from build123d import *

# Parameters (mm, degrees)
F0_R      = 15.625
F1_DEPTH  = 4
F2_R      = 2.45
F3_DEPTH  = 2
F4_R      = 3
F5_DEPTH  = 9.1
F6_R      = 1.55
F7_DEPTH  = 6
F8_R      = 5.5
F9_DEPTH  = 1
F11_R     = 0.5
F12_DEPTH = 1
F13_R     = 2
F14_DEPTH = 25.4


# Not quite as in the source:
# - a fillet or chamfer that OpenCascade refuses, or shapes differently, is made with other operations: its cross-section is extruded or revolved along the edge and cut away or added


with BuildPart() as f1:
    # F0 (on Front) → F1 (new body)
    with BuildSketch(Plane.XZ):
        Circle(F0_R)
    extrude(amount=F1_DEPTH)

    # F2 (on face) → F3 (join)
    with BuildSketch(Plane.XZ.offset(4)):
        Circle(F2_R)
    extrude(amount=F3_DEPTH)

    # F4 (on face) → F5 (join)
    with BuildSketch(Plane(origin=(0, 0, 0), x_dir=(-1, 0, 0), z_dir=(0, 1, 0))):
        Circle(F4_R)
    extrude(amount=F5_DEPTH)

    # F6 (on face) → F7 (cut)
    with BuildSketch(Plane(origin=(0, 9.1, 0), x_dir=(-1, 0, 0), z_dir=(0, 1, 0))):
        Circle(F6_R)
    extrude(amount=-F7_DEPTH, mode=Mode.SUBTRACT)

    # F8 (on face) → F9 (join)
    with BuildSketch(Plane.XZ.offset(4)):
        Circle(F8_R)
    extrude(amount=F9_DEPTH)

    # F10: fillet of radius 1.5875 on 3 edges, made by hand

    # F10_s1 → F10_t2 (revolve, cut)
    with BuildSketch(Plane.XY):
        with BuildLine():
            ThreePointArc((15.625, -2.4125), (15.1600320151, -3.5350320151), (14.0375, -4))
            Line((14.0375, -4), (15.625, -4))
            Line((15.625, -4), (15.625, -2.4125))
        make_face()
    revolve(axis=Axis((0, -4, 0), (0, -1, 0)), mode=Mode.SUBTRACT)

    # F10_s3 → F10_t4 (revolve, cut)
    with BuildSketch(Plane.XY):
        with BuildLine():
            ThreePointArc((15.625, -1.5875), (15.1600320151, -0.4649679849), (14.0375, 0))
            Line((14.0375, 0), (15.625, 0))
            Line((15.625, 0), (15.625, -1.5875))
        make_face()
    revolve(axis=Axis((0, 0, 0), (0, -1, 0)), mode=Mode.SUBTRACT)

    # F10_s5 → F10_t6 (revolve, cut)
    with BuildSketch(Plane.XY):
        with BuildLine():
            ThreePointArc((5.5, -4), (4.9161383637, -4.7264277948), (4.0252118796, -5))
            Line((4.0252118796, -5), (5.5, -5))
            Line((5.5, -5), (5.5, -4))
        make_face()
    revolve(axis=Axis((0, -5, 0), (0, -1, 0)), mode=Mode.SUBTRACT)

    # F11 (on face) → F12 (join)
    with BuildSketch(Plane.XZ.offset(5)):
        with Locations((-2.9818608891, 0.9871639777)):
            Circle(F11_R)
        with Locations((-2.258730121, 2.6503647678)):
            Circle(F11_R)
        with Locations((1.9354285905, 2.7226777747)):
            Circle(F11_R)
        with Locations((3.0201247428, 0.9510074742)):
            Circle(F11_R)
        with Locations((2.0800547209, -2.4115508422)):
            Circle(F11_R)
        with Locations((0, -3.2431513537)):
            Circle(F11_R)
        with Locations((-2.0779473707, -2.628490096)):
            Circle(F11_R)
    extrude(amount=F12_DEPTH)

    # F13 (on face) → F14 (cut)
    with BuildSketch(Plane.XZ.offset(4)):
        with Locations((-5.1422282122, 8.9166210964)):
            Circle(F13_R)
        with Locations((2.720073564, 9.3627097085)):
            Circle(F13_R)
        with Locations((7.9616084695, 3.7308477331)):
            Circle(F13_R)
        with Locations((7.6270420104, -3.2950392924)):
            Circle(F13_R)
        with Locations((2.9431174044, -8.0904858187)):
            Circle(F13_R)
        with Locations((-4.5288573019, -8.0347247422)):
            Circle(F13_R)
        with Locations((-8.9897383004, -3.1277562957)):
            Circle(F13_R)
        with Locations((-9.6588702872, 3.3405206632)):
            Circle(F13_R)
    extrude(amount=-F14_DEPTH, mode=Mode.SUBTRACT)


solid = f1.part
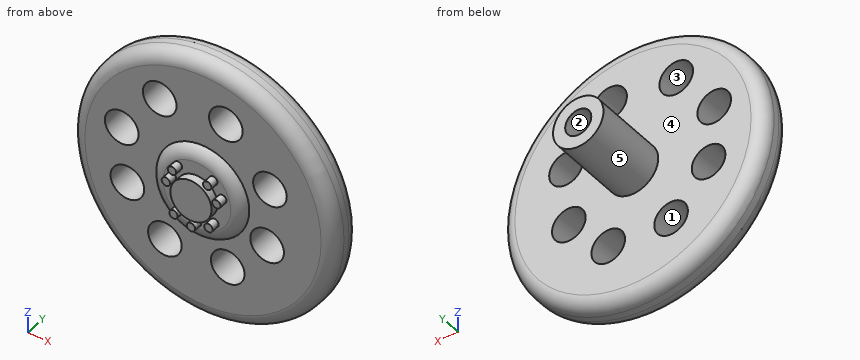
Here's how the part is built. I have some questions about the finished solid (model axes, mm). Face numbers are marked on the shaded views. A direction names the side the tool comes from. Round coordinates to 2 decimals unless told otherwise and drop trailing zeros. Loops run counter-clockwise (first coordinate to the right, second up) from the corner with the lowest first, then second, coordinate; pieces in that order, holes last. Notation, with made-up numbers: M 67.25,35.25 L 76.25,35.25 A21 cw 76.25,71.25 Z; hole C 59.5,63.5 d8. An arc over 180 degrees is marked long. Write each question's results on one line, items separated by ' | '. Start each with the question number.
(1) I want a section at B-B (y = 7.75). Please give me the cut outline in (x, z), then the cut area to 3 significant figures.
(2) Will these pins go through, and if not, where does the flat tip stop? P1, Ø6, axis at x = -5, y = -0.5, coming from the +Z side; P2, Ø8, axis at x = 3.5, z = -8.5, coming from the -Y side; P3, Ø0.9, axis at x = 0.5, z = -0.5, coming from the +Y side; P4, Ø8.5, axis at x = -7, z = 0, coming from the -Y side.
(3) If I drill on probe 1 along X at (y, z) = (-0.5, 2.5); probe 2 along X at (y, z) = (-3, 9); probe 3 along Y at (x, z) = (-13, -5), over which ranges is the centre line in solid material (lowest first)? Write a range as from..to.
(4) Thinking about a two-plate mould opening in X: for the marked faces 3, 4 and 5, which applies, pulls with the +X half, pulls with the -X half, needs draft (parallel to the pull), parting line crosses it, or undercut?
(5) I want a section at D-D (x = -8.5). State how many separate pieces and enclosed holes the cut face has, then the cut area to 3 significant figures.
(6) On a 3-axis mill with a long thin cutter (end or side, diameter ignored), from which of +Z, -Z, +X, -X, +Y, -Y can I reach the whole of each face in a straight line? I mean the marked faces 1 and 2. Say none if no direction works.
Solved:
1) outline: C 0,0 d6; hole C 0,0 d3.1 | area: 20.7 mm²
2) P1: stops at z = 15.47 | P2: stops at y = -4.49 | P3: stops at y = 3.1 | P4: stops at y = -6
3) probe 1: x = -14.99..-11.47, -7.84..6.39, 9.54..14.99 | probe 2: x = -12.63..-7.14, -3.14..0.75, 4.69..12.63 | probe 3: y = -4..0
4) face 3: undercut | face 4: needs draft | face 5: parting line crosses it
5) separate pieces: 3 | enclosed holes: 0 | area: 73.7 mm²
6) face 1: +Y, -Y | face 2: +Y
